Input: part model. Units: mm. Frame: model coordinates. Face numbers are marked on the shaded views. Give positions to 0.01 mm unless a question says otherwise; leave off trailing zeros. Order: outer loops, then holes, each group sorted by start corner. A loop starts at its lowest first (then second) coordinate and runs counter-clockwise, first axis right, second up. Notation, with made-up numbers: M 50.5,49 L 96.5,49 A11 cw 96.5,56 Z; hole C 11,73 d7. An arc over 180 degrees is marked long. Use a Markdown table: item, result.
from build123d import *

# Parameters (mm, degrees)
SKETCH1_W             = 110.5
SKETCH1_H             = 72.2
SKETCH1_W_2           = 106.5
SKETCH1_H_2           = 68.2
BOSS_EXTRUDE1_DEPTH   = 5
BOSS_EXTRUDE2_DEPTH   = 2
SKETCH4_R             = 12.75
SKETCH4_R_2           = 10.75
BOSS_EXTRUDE3_DEPTH   = 2
BOSS_EXTRUDE3_2_DEPTH = 2
SKETCH5_R             = 10.75
SKETCH5_W             = 106.5
SKETCH5_H             = 68.2
SKETCH5_W_2           = 10
SKETCH5_H_2           = 20
BOSS_EXTRUDE4_DEPTH   = 2


with BuildPart() as part:
    # Sketch1 → Boss-Extrude1 (new body)
    with BuildSketch(Plane(origin=(0, 8.5, 0), x_dir=(1, 0, 0), z_dir=(0, 1, 0))):
        Rectangle(SKETCH1_W, SKETCH1_H)
        Rectangle(SKETCH1_W_2, SKETCH1_H_2, mode=Mode.SUBTRACT)
    extrude(amount=BOSS_EXTRUDE1_DEPTH)

    # Sketch2 → Boss-Extrude2 (add)
    with BuildSketch(Plane(origin=(0, 8.5, 0), x_dir=(1, 0, 0), z_dir=(0, 1, 0))):
        Polygon((-55.25, 36.1), (-55.25, -36.1), (-48.25, -36.1), (-48.25, -30.1), (-49.25, -30.1), (-49.25, 30.1), (-18.75, 30.1), (-18.75, 36.1), align=None)
        Polygon((55.25, -36.1), (55.25, 36.1), (48.25, 36.1), (48.25, 30.1), (49.25, 30.1), (49.25, -30.1), (18.75, -30.1), (18.75, -36.1), align=None)
    extrude(amount=-BOSS_EXTRUDE2_DEPTH)



with BuildPart() as body_2:
    # Sketch4 → Boss-Extrude3 (new body)
    with BuildSketch(Plane(origin=(0, 13, 0), x_dir=(1, 0, 0), z_dir=(0, 1, 0))):
        with Locations(Location((-43.5, 60, 0), (0, 0, 270))):
            Circle(SKETCH4_R)
        with Locations(Location((-43.5, 60, 0), (0, 0, 270))):
            Circle(SKETCH4_R_2, mode=Mode.SUBTRACT)
    extrude(amount=BOSS_EXTRUDE3_DEPTH)


with BuildPart() as body_3:
    # Sketch4 → Boss-Extrude3 2 (new body)
    with BuildSketch(Plane(origin=(0, 13, 0), x_dir=(1, 0, 0), z_dir=(0, 1, 0))):
        with Locations(Location((43.5, 60, 0), (0, 0, 270))):
            Circle(SKETCH4_R)
        with Locations(Location((43.5, 60, 0), (0, 0, 270))):
            Circle(SKETCH4_R_2, mode=Mode.SUBTRACT)
    extrude(amount=BOSS_EXTRUDE3_2_DEPTH)


with BuildPart() as part_1:
    add(part.part)

    add(body_2.part)  # Boss-Extrude4 merges body 2

    add(body_3.part)  # Boss-Extrude4 merges body 3
    # Sketch5 → Boss-Extrude4 (add)
    with BuildSketch(Plane(origin=(0, 13, 0), x_dir=(1, 0, 0), z_dir=(0, 1, 0))):
        Polygon((-56.5, -35), (-56.5, 79), (-43.619883045, 83.687979185), (-40, 82), (40, 82), (43.619883045, 83.687979185), (56.5, 79), (56.5, -35), (55, -37), (-55, -37), align=None)
        with Locations(Location((-43.5, 60, 0), (0, 0, 270))):
            Circle(SKETCH5_R, mode=Mode.SUBTRACT)
        with Locations(Location((43.5, 60, 0), (0, 0, 270))):
            Circle(SKETCH5_R, mode=Mode.SUBTRACT)
        Rectangle(SKETCH5_W, SKETCH5_H, mode=Mode.SUBTRACT)
        with Locations((0, 52)):
            Rectangle(SKETCH5_W_2, SKETCH5_H_2, mode=Mode.SUBTRACT)
    extrude(amount=-BOSS_EXTRUDE4_DEPTH)


solid = part_1.part
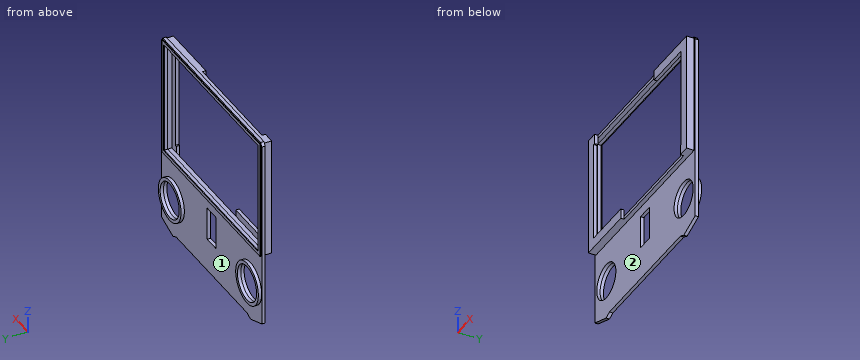
1) Cut plane B-B on x = -8. Return loops of the section in (y, z), and give its area (3 significant figures).
Response values:
| item | result |
|---|---|
| outline | M 8.5,-36.1 L 11,-36.1 L 11,-82 L 13,-82 L 13,-36.1 L 13.5,-36.1 L 13.5,-34.1 L 8.5,-34.1 Z; M 8.5,34.1 L 13.5,34.1 L 13.5,36.1 L 13,36.1 L 13,37 L 11,37 L 11,36.1 L 8.5,36.1 Z |
| area | 114 mm² |
2) Mould query, pull axis Z, two halves, no side actions, for the marked faces 1 and 2. Classes: released by +Z, released by -Z, zero draft, split by the parting line, or undercut.
Response values:
| item | result |
|---|---|
| face 1 | undercut |
| face 2 | zero draft |
3) Cut plane C-C on z = -60. Return loops of the section in (x, y), and give its area (3 significant figures).
Response values:
| item | result |
|---|---|
| outline | M -56.5,11 L -54.25,11 L -54.25,15 L -56.25,15 L -56.25,13 L -56.5,13 Z; M -32.75,11 L -5,11 L -5,13 L -30.75,13 L -30.75,15 L -32.75,15 Z; M 5,11 L 32.75,11 L 32.75,15 L 30.75,15 L 30.75,13 L 5,13 Z; M 54.25,11 L 56.5,11 L 56.5,13 L 56.25,13 L 56.25,15 L 54.25,15 Z |
| area | 136 mm² |
4) First-contact query: pin 1 Ø5 at (x, y) = (-36, 11) entering from -Z; pin 2 Ø1 at (y, z) = (8, 1.5) entering from -X; pin 3 Ø1.5 at (x, y) = (-44, 10) entering from +Z. Flat tips, straight axial feed; report the tip coordinate or a pass-through.
Response values:
| item | result |
|---|---|
| pin 1 | stops at z = -82 |
| pin 2 | stops at x = -55.25 |
| pin 3 | stops at z = 36.1 |
5) Cut plane D-D on x = 29. Return loops of the section in (y, z), and give its area (3 significant figures).
Response values:
| item | result |
|---|---|
| outline | M 6.5,30.1 L 8.5,30.1 L 8.5,34.1 L 13.5,34.1 L 13.5,36.1 L 13,36.1 L 13,37 L 11,37 L 11,36.1 L 6.5,36.1 Z; M 8.5,-36.1 L 11,-36.1 L 11,-82 L 13,-82 L 13,-36.1 L 13.5,-36.1 L 13.5,-34.1 L 8.5,-34.1 Z |
| area | 126 mm² |
6) Material intervals for line 1 (X direction, y = 12.1, z = -60); line 2 (X direction, y = 13.5, z = -60); line 3 (Z direction, x = 15.5, y = 10.5), sorted ascending. Write a range as from..to.
Response values:
| item | result |
|---|---|
| line 1 | x = -56.5..-54.25, -32.75..-5, 5..32.75, 54.25..56.5 |
| line 2 | x = -56.25..-54.25, -32.75..-30.75, 30.75..32.75, 54.25..56.25 |
| line 3 | z = -36.1..-34.1, 34.1..36.1 |
7) Cut plane A-A on z = -11. Return loops of the section in (x, y), and give its area (3 significant figures).
Response values:
| item | result |
|---|---|
| outline | M -56.5,11 L -55.25,11 L -55.25,6.5 L -49.25,6.5 L -49.25,8.5 L -53.25,8.5 L -53.25,13.5 L -55.25,13.5 L -55.25,13 L -56.5,13 Z; M 49.25,6.5 L 55.25,6.5 L 55.25,11 L 56.5,11 L 56.5,13 L 55.25,13 L 55.25,13.5 L 53.25,13.5 L 53.25,8.5 L 49.25,8.5 Z |
| area | 49.0 mm² |
